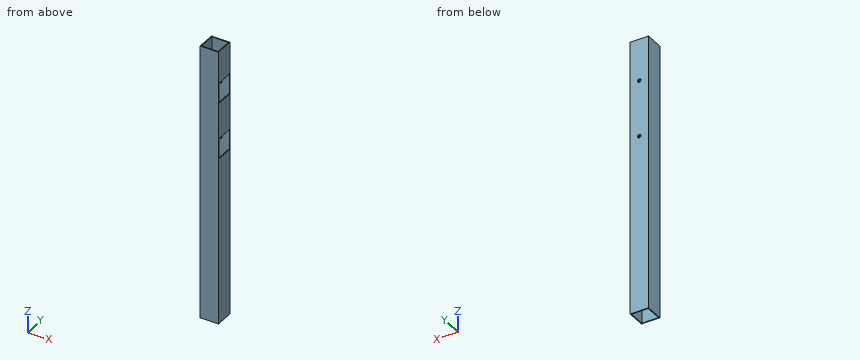
from build123d import *

# Parameters (mm, degrees)
F0_W      = 63.5
F0_H      = 63.5
F0_W_2    = 57.5
F0_H_2    = 57.5
F1_DEPTH  = 950
F2_W      = 57.5
F2_H      = 70
F3_DEPTH  = 3
F4_W      = 57.5
F4_H      = 70
F5_DEPTH  = 3
F7_DEPTH  = 3
F8_DEPTH  = 3
F9_R      = 6
F10_DEPTH = 3
F11_R     = 6
F12_DEPTH = 3


with BuildPart() as f1:
    # F0 (on Top) → F1 (new body)
    with BuildSketch(Plane.XY):
        with Locations((7.6151648536, -5.7103513741)):
            Rectangle(F0_W, F0_H)
        with Locations((7.6151648536, -5.7103513741)):
            Rectangle(F0_W_2, F0_H_2, mode=Mode.SUBTRACT)
    extrude(amount=F1_DEPTH)

    # F2 (on face) → F3 (cut)
    with BuildSketch(Plane.YZ.offset(39.3651648536)):
        with Locations((-5.7103513741, 805)):
            Rectangle(F2_W, F2_H)
    extrude(amount=-F3_DEPTH, mode=Mode.SUBTRACT)

    # F4 (on face) → F5 (cut)
    with BuildSketch(Plane.YZ.offset(39.3651648536)):
        with Locations((-5.7103513741, 611)):
            Rectangle(F4_W, F4_H)
    extrude(amount=-F5_DEPTH, mode=Mode.SUBTRACT)

    # F9 (on face) → F10 (cut)
    with BuildSketch(Plane(origin=(0, 26.0396486259, 0), x_dir=(-1, 0, 0), z_dir=(0, 1, 0))):
        with Locations((-7.6151648536, 805)):
            Circle(F9_R)
    extrude(amount=-F10_DEPTH, mode=Mode.SUBTRACT)

    # F11 (on face) → F12 (cut)
    with BuildSketch(Plane(origin=(0, 26.0396486259, 0), x_dir=(-1, 0, 0), z_dir=(0, 1, 0))):
        with Locations((-7.6151648536, 611)):
            Circle(F11_R)
    extrude(amount=-F12_DEPTH, mode=Mode.SUBTRACT)


with BuildPart() as f7:
    # F4 (on face) → F7 (new body)
    with BuildSketch(Plane.YZ.offset(39.3651648536)):
        with Locations((-5.7103513741, 611)):
            Rectangle(F4_W, F4_H)
    extrude(amount=F7_DEPTH)

    # F8 (cut): a face of the model
    f8_faces = [f7.faces().sort_by_distance(p)[0] for p in [
        (42.3651648536, -5.7103513741, 611),
    ]]
    extrude(f8_faces, amount=-F8_DEPTH, mode=Mode.SUBTRACT)


solid = f1.part
Read the model definition and answer for the solid it produces. Units are mm, in the model's axes. Round coordinates to 2 decimals unless told otherwise and drop trailing zeros. Write each loop counter-clockwise with the first axis right and the second up, starting at its lowest first coordinate (ties: lowest second). Pieces come first, ordered by that corner, then holes.
Q1. Find section A-A on z = 394. Determine the outline of the cut face in (x, y), and give its area (3 significant figures).
Values:
outline: (-24.13, -37.46) - (39.37, -37.46) - (39.37, 26.04) - (-24.13, 26.04) - close; hole (-21.13, -34.46) - (36.37, -34.46) - (36.37, 23.04) - (-21.13, 23.04) - close
area: 726 mm2
Q2. Find section D-D on z = 633.5. Determine the outline of the cut face in (x, y), and give its area (4 significant figures).
Values:
outline: (-24.13, -37.46) - (39.37, -37.46) - (39.37, -34.46) - (-21.13, -34.46) - (-21.13, 23.04) - (39.37, 23.04) - (39.37, 26.04) - (-24.13, 26.04) - close
area: 553.5 mm2
Q3. Straight lines are drawn through the part: line 1 (Y direction, x = 29.5, z = 74.5); line 2 (X direction, y = -14.5, z = 754); line 3 (X direction, y = 25.25, z = 611). For each, find the intervals that lie inside material, in ascending order.
Values:
line 1: y = -37.46 to -34.46, 23.04 to 26.04
line 2: x = -24.13 to -21.13, 36.37 to 39.37
line 3: x = -24.13 to 1.62, 13.62 to 39.37
Q4. Find section B-B on x = 25. Determine the outline of the cut face in (y, z), and give its area (3 significant figures).
Values:
outline: (-37.46, 0) - (-34.46, 0) - (-34.46, 950) - (-37.46, 950) - close; (23.04, 0) - (26.04, 0) - (26.04, 950) - (23.04, 950) - close
area: 5,700 mm2
Q5. Find section C-C on y = -23.5. Determine the outline of the cut face in (x, z).
Values:
outline: (-24.13, 0) - (-21.13, 0) - (-21.13, 950) - (-24.13, 950) - close; (36.37, 0) - (39.37, 0) - (39.37, 576) - (36.37, 576) - close; (36.37, 646) - (39.37, 646) - (39.37, 770) - (36.37, 770) - close; (36.37, 840) - (39.37, 840) - (39.37, 950) - (36.37, 950) - close
